from build123d import *

# Parameters (mm, degrees)
F1_DEPTH = 20
F2_SIZE2 = 7
F2_SIZE  = 8
F3_R     = 3


with BuildPart() as f1:
    # F0 (on Top) → F1 (new body)
    with BuildSketch(Plane.XY):
        with BuildLine():
            ThreePointArc((2, 5.9741108125), (5.1132181647, 3.6803532439), (6.3, 0))
            ThreePointArc((6.3, 0), (5.1132181647, -3.6803532439), (2, -5.9741108125))
            Line((2, -5.9741108125), (2, -9.7979589711))
            ThreePointArc((2, -9.7979589711), (7.7459666924, -6.3245553203), (10, 0))
            ThreePointArc((10, 0), (7.7459666924, 6.3245553203), (2, 9.7979589711))
            Line((2, 9.7979589711), (2, 5.9741108125))
        make_face()
        with BuildLine():
            ThreePointArc((-2, 5.9741108125), (0, 6.3), (2, 5.9741108125))
            Line((2, 5.9741108125), (2, 9.7979589711))
            ThreePointArc((2, 9.7979589711), (0, 10), (-2, 9.7979589711))
            Line((-2, 9.7979589711), (-2, 5.9741108125))
        make_face()
        with BuildLine():
            ThreePointArc((-2, -5.9741108125), (-6.3, 0), (-2, 5.9741108125))
            Line((-2, 5.9741108125), (-2, 9.7979589711))
            ThreePointArc((-2, 9.7979589711), (-10, 0), (-2, -9.7979589711))
            Line((-2, -9.7979589711), (-2, -5.9741108125))
        make_face()
        with BuildLine():
            Line((2, -9.7979589711), (2, -5.9741108125))
            ThreePointArc((2, -5.9741108125), (0, -6.3), (-2, -5.9741108125))
            Line((-2, -5.9741108125), (-2, -9.7979589711))
            ThreePointArc((-2, -9.7979589711), (0, -10), (2, -9.7979589711))
        make_face()
        with BuildLine():
            Line((2, -30.2020410289), (2, -9.7979589711))
            ThreePointArc((2, -9.7979589711), (0, -10), (-2, -9.7979589711))
            Line((-2, -9.7979589711), (-2, -40))
            ThreePointArc((-2, -40), (-0.9614813968, -34.7084973779), (2, -30.2020410289))
        make_face()
        with BuildLine():
            Line((2, -40), (2, -30.2020410289))
            ThreePointArc((2, -30.2020410289), (-0.9614813968, -34.7084973779), (-2, -40))
            Line((-2, -40), (2, -40))
        make_face()
        with BuildLine():
            Line((2, -40), (-2, -40))
            ThreePointArc((-2, -40), (12, -54), (26, -40))
            ThreePointArc((26, -40), (23.8321595662, -32.5166852265), (18, -27.3508893593))
            Line((18, -27.3508893593), (16.2857142857, -30.9649209709))
            ThreePointArc((16.2857142857, -30.9649209709), (20.4515425473, -34.6547751618), (22, -40))
            ThreePointArc((22, -40), (12, -50), (2, -40))
        make_face()
    extrude(amount=F1_DEPTH)

    # F2
    f2_edges = [f1.edges().sort_by_distance(p)[0] for p in [
        (17.142857, -29.157905, 20),
        (17.142857, -29.157905, 0),
    ]]
    f2_side = f1.faces().sort_by_distance((17.142857, -29.157905, 10))[0]
    chamfer(f2_edges, length=F2_SIZE, length2=F2_SIZE2, reference=f2_side)

    # F3
    f3_edges = [f1.edges().sort_by_distance(p)[0] for p in [
        (17.142857, -29.157905, 12),
        (17.142857, -29.157905, 8),
    ]]
    fillet(f3_edges, radius=F3_R)


solid = f1.part
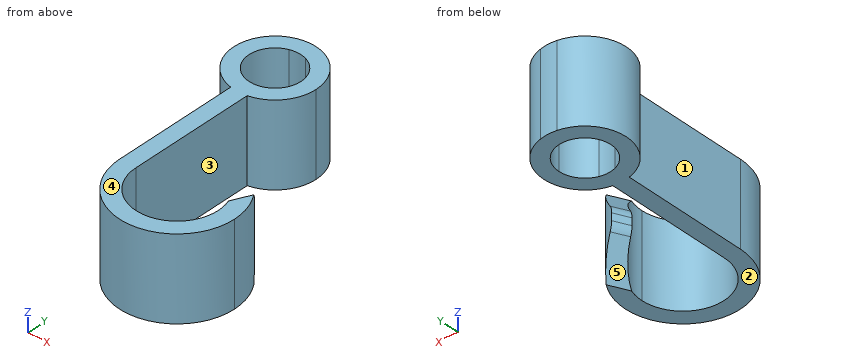
Design review of the part built by this model. Coordinates are the model's own, in mm. Face numbers are marked on the shaded views. A direction names the side the tool comes from. Round coordinates to 2 decimals unless told otherwise and drop trailing zeros. Write each loop counter-clockwise with the first axis right and the second up, starting at its lowest first coordinate (ties: lowest second). Pieces come first, ordered by that corner, then holes. Notation, with made-up numbers: M -40,-6.75 L -2,-6.75 A13 cw -2,18.25 Z; hole C -2.5,-14 d3. An arc over 180 degrees is marked long. One line per item, written item: value. Start each with the question number.
1. Take a section at D-D on z = 2.5. State the section outline as (x, y) points.
2. Clearance check with flat-ended pins moving along their axes: P1, Ø1.5, axis at x = 4, z = 15.5, coming from the -Y side; P2, Ø1, axis at y = 0.5, z = 15.5, coming from the +X side; P3, Ø1.5, axis at x = -3, z = 9, coming from the +Y side. State where each tip first meets the part, or that it passes through.
3. For the marked faces 4 and 5, list the 3-axis set-ups (+Z, -Z, +X, -X, +Y, -Y) from which the entire face can be reached by the end or side of a thin tool; tool diameter is ignored.
4. To check wall thickness, follow probe 1 along X at (y, z) = (-40.5, 3.75); probe 2 along X at (y, z) = (2, 15); probe 3 along X at (y, z) = (-21, 12.5). State the ranges of each line that lie inside material, in increasing order. Write a range as from..to.
5. Take a section at B-B on x = 4. State the section outline as (y, z) points.
6. Take a section at A-A on y = -48. State the section outline as (x, z) points, then the cut area to 3 significant figures.
7. Draft analysis for pull direction X (two halves, no side actions). For the marked faces 1, 2 and 3, state which applies: pulls with the +X half, pulls with the -X half, needs draft (parallel to the pull), parting line crosses it, or undercut.
8. Take a section at C-C on z = 11.5. State the section outline as (x, y) points.
Computed:
1. outline: M -2,-40 A14 ccw long 21.98,-30.18 L 20.1,-34.14 A10 cw long 2,-40 L 2,-9.8 A10 ccw long -2,-9.8 Z; hole C 0,0 d12.6
2. P1: stops at y = -51.98
2. P2: stops at x = 10
2. P3: stops at y = 9.74
3. face 4: +Z, +X, -X, +Y, -Y
3. face 5: -Z, +Y
4. probe 1: x = -1.99..2.01, 21.99..25.99
4. probe 2: x = -9.8..-5.97, 5.97..9.8
4. probe 3: x = -2..2
5. outline: M -51.49,0 L -46,0 L -46,20 L -51.49,20 Z; M -9.17,0 L -4.87,0 L -4.87,20 L -9.17,20 Z; M 4.87,0 L 9.17,0 L 9.17,20 L 4.87,20 Z
6. outline: M 0.51,0 L 6,0 L 6,20 L 0.51,20 Z; M 18,0 L 23.49,0 L 23.49,20 L 18,20 Z
6. area: 220 mm²
7. face 1: pulls with the -X half
7. face 2: needs draft
7. face 3: undercut
8. outline: M -2,-40 A14 ccw long 18.06,-27.38 L 16.35,-30.99 A10 cw long 2,-40 L 2,-9.8 A10 ccw long -2,-9.8 Z; hole C 0,0 d12.6
